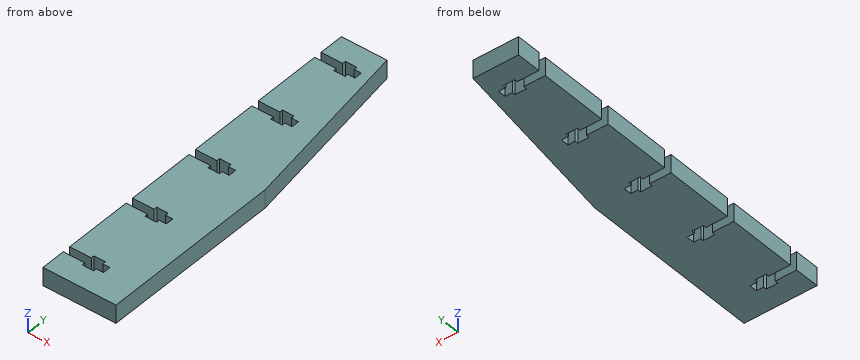
from build123d import *

# Parameters (mm, degrees)
SKETCH1_W               = 6.35
SKETCH1_H               = 127
BOSS_EXTRUDE1_DEPTH     = 25.4
CUT_EXTRUDE1_DEPTH      = 69.685751798
CUT_EXTRUDE1_DEPTH_BACK = 69.685751798


with BuildPart() as part:
    # Sketch1 → Boss-Extrude1 (new body)
    with BuildSketch(Plane(origin=(0, 0, 0), x_dir=(0, 0, -1), z_dir=(1, 0, 0))):
        Rectangle(SKETCH1_W, SKETCH1_H)
    extrude(amount=BOSS_EXTRUDE1_DEPTH)

    # Sketch4 → Cut-Extrude1 (cut, two sides: drawn at the far end of the back side and taken through both)
    with BuildSketch(Plane.XY.offset(3.175).offset(-CUT_EXTRUDE1_DEPTH_BACK)):
        Polygon((7.5, 54.875), (0, 54.875), (0, 52.125), (7.5, 52.125), (7.5, 51), (11.5, 51), (11.5, 52.125), (14, 52.125), (14, 54.875), (11.5, 54.875), (11.5, 56), (7.5, 56), align=None)
        Polygon((25.4, 63.5), (15.875, 63.5), (25.4, 0), align=None)
        Polygon((7.5, 28.125), (0, 28.125), (0, 25.375), (7.5, 25.375), (7.5, 24.25), (11.5, 24.25), (11.5, 25.375), (14, 25.375), (14, 28.125), (11.5, 28.125), (11.5, 29.25), (7.5, 29.25), align=None)
        Polygon((7.5, 1.375), (0, 1.375), (0, -1.375), (7.5, -1.375), (7.5, -2.5), (11.5, -2.5), (11.5, -1.375), (14, -1.375), (14, 1.375), (11.5, 1.375), (11.5, 2.5), (7.5, 2.5), align=None)
        Polygon((7.5, -25.375), (0, -25.375), (0, -28.125), (7.5, -28.125), (7.5, -29.25), (11.5, -29.25), (11.5, -28.125), (14, -28.125), (14, -25.375), (11.5, -25.375), (11.5, -24.25), (7.5, -24.25), align=None)
        Polygon((7.5, -52.125), (0, -52.125), (0, -54.875), (7.5, -54.875), (7.5, -56), (11.5, -56), (11.5, -54.875), (14, -54.875), (14, -52.125), (11.5, -52.125), (11.5, -51), (7.5, -51), align=None)
    extrude(amount=CUT_EXTRUDE1_DEPTH + CUT_EXTRUDE1_DEPTH_BACK, mode=Mode.SUBTRACT)


solid = part.part
Work out the finished part from the listing and answer in its coordinate system (mm). Coordinates: 2 decimals unless noted, no trailing zeros. Write each loop counter-clockwise with the first axis right and the second up, starting at its lowest first coordinate (ties: lowest second). Pieces come first, ordered by that corner, then holes.
1. The part is cut by section B-B, the plane x = 3.25. Write down the section's boundary in (y, z) (3 decimals).
Results list:
outline: (-63.5, -3.175) - (-54.875, -3.175) - (-54.875, 3.175) - (-63.5, 3.175) - close; (-52.125, -3.175) - (-28.125, -3.175) - (-28.125, 3.175) - (-52.125, 3.175) - close; (-25.375, -3.175) - (-1.375, -3.175) - (-1.375, 3.175) - (-25.375, 3.175) - close; (1.375, -3.175) - (25.375, -3.175) - (25.375, 3.175) - (1.375, 3.175) - close; (28.125, -3.175) - (52.125, -3.175) - (52.125, 3.175) - (28.125, 3.175) - close; (54.875, -3.175) - (63.5, -3.175) - (63.5, 3.175) - (54.875, 3.175) - close
2. Consider line 1 along Y through (x, z) = (3.75, 1.5) (3 decimals); line 2 along Y through (x, z) = (8.5, -0.75); line 3 along X through (y, z) = (29, 0.25). Determine where each line is inside the solid, lowest interval first.
Results list:
line 1: y = -63.5 to -54.875, -52.125 to -28.125, -25.375 to -1.375, 1.375 to 25.375, 28.125 to 52.125, 54.875 to 63.5
line 2: y = -63.5 to -56, -51 to -29.25, -24.25 to -2.5, 2.5 to 24.25, 29.25 to 51, 56 to 63.5
line 3: x = 0 to 7.5, 11.5 to 21.05
3. The part is cut by section A-A, the plane x = 9. Write down the section's boundary in (y, z) (3 decimals), and give its area (3 significant figures).
Results list:
outline: (-63.5, -3.175) - (-56, -3.175) - (-56, 3.175) - (-63.5, 3.175) - close; (-51, -3.175) - (-29.25, -3.175) - (-29.25, 3.175) - (-51, 3.175) - close; (-24.25, -3.175) - (-2.5, -3.175) - (-2.5, 3.175) - (-24.25, 3.175) - close; (2.5, -3.175) - (24.25, -3.175) - (24.25, 3.175) - (2.5, 3.175) - close; (29.25, -3.175) - (51, -3.175) - (51, 3.175) - (29.25, 3.175) - close; (56, -3.175) - (63.5, -3.175) - (63.5, 3.175) - (56, 3.175) - close
area: 648 mm2
4. The part is cut by section C-C, the plane x = 24. Write down the section's boundary in (y, z) (3 decimals), and give its area (3 significant figures).
Results list:
outline: (-63.5, -3.175) - (9.333, -3.175) - (9.333, 3.175) - (-63.5, 3.175) - close
area: 462 mm2
5. Flat-ended cylindrical pins translate along their axes: pin 1 (1.5 mm diameter, centred on y = 45.5, z = 2.5, fed in from +X); pin 2 (1.2 mm diameter, centred on y = 55.5, z = 1.5, fed in from +X) (3 decimals). Find the tip coordinate at first contact, or state that the pin passes through.
Results list:
pin 1: stops at x = 18.69
pin 2: stops at x = 17.165
